```python
from build123d import *

# Parameters (mm, degrees)
PAD_DEPTH       = 20
THICKNESS_T     = 2
SKETCH001_W     = 15
SKETCH001_H     = 2
PAD001_DEPTH    = 6
SKETCH002_R     = 1.4
POCKET_DEPTH    = 2.001
SKETCH003_W     = 15
SKETCH003_H     = 2
PAD002_DEPTH    = 6
SKETCH004_R     = 1.4
POCKET001_DEPTH = 22.001
SKETCH005_R     = 1.6
POCKET002_DEPTH = 22.001
SKETCH006_W     = 7
SKETCH006_H     = 4
POCKET003_DEPTH = 2


with BuildPart() as part:
    # Sketch → Pad (new body)
    with BuildSketch(Plane.XY):
        with BuildLine():
            Line((0, 37), (46, 37))
            ThreePointArc((49, 34), (48.1213203436, 36.1213203436), (46, 37))
            Line((49, 34), (49, 3))
            ThreePointArc((46, 0), (48.1213203436, 0.8786796564), (49, 3))
            Line((46, 0), (0, 0))
            ThreePointArc((-3, 3), (-2.1213203436, 0.8786796564), (0, 0))
            Line((-3, 3), (-3, 34))
            ThreePointArc((0, 37), (-2.1213203436, 36.1213203436), (-3, 34))
        make_face()
    extrude(amount=PAD_DEPTH)

    # Thickness
    thickness_openings = [part.faces().sort_by_distance(p)[0] for p in [
        (23, 18.5, 20),
    ]]
    offset(amount=THICKNESS_T, openings=thickness_openings, kind=Kind.INTERSECTION)

    # Sketch001 → Pad001 (new body)
    with BuildSketch(Plane(origin=(0, 39, 0), x_dir=(-1, 0, 0), z_dir=(0, 1, 0))):
        with Locations((-23, -1)):
            Rectangle(SKETCH001_W, SKETCH001_H)
    extrude(amount=PAD001_DEPTH)

    # Sketch002 → Pocket (cut, through all)
    with BuildSketch(Plane.XY):
        with Locations((23, 42)):
            Circle(SKETCH002_R)
    extrude(amount=-POCKET_DEPTH, mode=Mode.SUBTRACT)

    # Sketch003 → Pad002 (new body)
    with BuildSketch(Plane.XZ.offset(2)):
        with Locations((23, -1)):
            Rectangle(SKETCH003_W, SKETCH003_H)
    extrude(amount=PAD002_DEPTH)

    # Sketch004 → Pocket001 (cut, through all)
    with BuildSketch(Plane(origin=(0, 0, -2), x_dir=(1, 0, 0), z_dir=(0, 0, -1))):
        with Locations((23, 5)):
            Circle(SKETCH004_R)
    extrude(amount=-POCKET001_DEPTH, mode=Mode.SUBTRACT)

    # Sketch005 → Pocket002 (cut, through all)
    with BuildSketch(Plane(origin=(0, 0, -2), x_dir=(1, 0, 0), z_dir=(0, 0, -1))):
        with Locations((2, -17.739397)):
            Circle(SKETCH005_R)
        with Locations((44, -17.314964)):
            Circle(SKETCH005_R)
    extrude(amount=-POCKET002_DEPTH, mode=Mode.SUBTRACT)

    # Sketch006 → Pocket003 (cut)
    with BuildSketch(Plane.XZ.offset(2)):
        with Locations((22, 8)):
            Rectangle(SKETCH006_W, SKETCH006_H)
    extrude(amount=-POCKET003_DEPTH, mode=Mode.SUBTRACT)


solid = part.part
```
Can you work these out from the model? Positions are in its coordinate system, mm. A direction names the side the tool comes from. Give positions to 0.01 mm unless a question says otherwise; leave off trailing zeros. Loops run counter-clockwise (first coordinate to the right, second up) from the corner with the lowest first, then second, coordinate; pieces in that order, holes last. Notation, with made-up numbers: M 65.5,87.5 L 96.5,87.5 A26 cw 96.5,125.5 Z; hole C 6.25,47.5 d4. An arc over 180 degrees is marked long. One line per item, written item: value.
(1) I need wall thicknesses on line 1 (Y direction, x = 23, z = -1.5); line 2 (X direction, y = -5, z = -1.25); line 3 (X direction, y = 7, z = 4.25). Which ranges of each line are inside material? Lowest first, please.
Returned:
line 1: -8 to -6.4, -3.6 to 40.6, 43.4 to 45
line 2: 15.5 to 21.6, 24.4 to 30.5
line 3: -5 to -3, 49 to 51
(2) Suppose I cut it at B-B on x = 2. List the corners of the cut face in (y, z) for me.
Returned:
outline: M -2,-2 L 16.14,-2 L 16.14,0 L 0,0 L 0,20 L -2,20 Z; M 19.34,-2 L 39,-2 L 39,20 L 37,20 L 37,0 L 19.34,0 Z
(3) Suppose I cut it at D-D on z = 3.75. List the corners of the cut face in (x, y) for me, plus the area to 3 significant figures.
Returned:
outline: M -5,3 A5 ccw 0,-2 L 46,-2 A5 ccw 51,3 L 51,34 A5 ccw 46,39 L 0,39 A5 ccw -5,34 Z; hole M -3,3 A3 ccw 0,0 L 46,0 A3 ccw 49,3 L 49,34 A3 ccw 46,37 L 0,37 A3 ccw -3,34 Z
area: 358 mm^2
(4) Suppose I cut it at C-C on x = 14. List the corners of the cut face in (y, z) for me.
Returned:
outline: M -2,-2 L 39,-2 L 39,20 L 37,20 L 37,0 L 0,0 L 0,20 L -2,20 Z
(5) We'd pull the mould along Z, two halves only. Please class faces 4 (the face through (23, 19, 0)), 5 (the face through (22, -1, 6)), 6 (the face through (23, 37, 10)): released by +Z, released by -Z, zero draft, split by the parting line, or undercut.
Returned:
face 4: released by +Z
face 5: undercut
face 6: zero draft
(6) Which directions (+Z, -Z, +X, -X, +Y, -Y) give clear straight access to the entire face, cutting with the end or side of a thin tool? Please do faces 1 (the face through (25, -5, 0)), 2 (the face through (18.5, -1, 8)), 3 (the face through (15.5, -5, -1)).
Returned:
face 1: +Z, +X, -X, -Y
face 2: -Y
face 3: +Z, -Z, -X, -Y
(7) Suppose I cut it at A-A on y = -5. List the corners of the cut face in (x, z) for me.
Returned:
outline: M 15.5,-2 L 21.6,-2 L 21.6,0 L 15.5,0 Z; M 24.4,-2 L 30.5,-2 L 30.5,0 L 24.4,0 Z
(8) Will these pins go through, and if not, where does the flat tip stop? pin 1 (1.5 mm diameter, centred on x = 39, z = 13, fed in from -Y); pin 2 (1 mm diameter, centred on y = 41.5, z = -1, fed in from +X); pin 3 (6 mm diameter, centred on x = 15.5, y = 9, fed in from +Z); pin 4 (4 mm diameter, centred on y = 34.5, z = 6, fed in from +X).
Returned:
pin 1: y = -2
pin 2: x = 30.5
pin 3: z = 0
pin 4: x = 51
